Geometry check sheet. Reference: the model listing, model coordinates, mm. Face numbers are marked on the shaded views. A direction names the side the tool comes from. Give positions to 0.01 mm unless a question says otherwise; leave off trailing zeros. Loops run counter-clockwise (first coordinate to the right, second up) from the corner with the lowest first, then second, coordinate; pieces in that order, holes last. Notation, with made-up numbers: (36, -38.75) -> (75, -38.75) arc R24 cw to (75, -1.75) -> close; hole circle Ø3 at (-8, 68.5). An arc over 180 degrees is marked (long way). One line per question, with ' | ' between items.
from build123d import *

# Parameters (mm, degrees)
SKETCH_1_W           = 50
SKETCH_1_H           = 40
EXTRUDE_1_DEPTH      = 4
SKETCH_2_R           = 2
CUT_EXTRUDE_1_DEPTH  = 4
EXTRUDE_2_DEPTH      = 180
CUT_EXTRUDE_START    = -60
CUT_EXTRUDE_2_DEPTH  = 60
CUT_EXTRUDE_3_DEPTH  = 60
EXTRUDE_3_REACH      = 191.95
EXTRUDE_3_END_RADIUS = 230
EXTRUDE_START        = 38
EXTRUDE_4_DEPTH      = 38
CUT_EXTRUDE_4_DEPTH  = 211.154705038
SKETCH_9_R           = 3.5
EXTRUDE_5_DEPTH      = 40
SKETCH_10_R          = 1.5
CUT_EXTRUDE_5_DEPTH  = 30
CHAMFER_1_SIZE       = 0.5
EXTRUDE_6_REACH      = 171.111
EXTRUDE_6_END_RADIUS = 235
EXTRUDE_7_REACH      = 171.111


with BuildPart() as part:
    # 草图1 → 凸台-拉伸1 (new body)
    with BuildSketch(Plane(origin=(0, 0, 0), x_dir=(0, 0, -1), z_dir=(1, 0, 0))):
        with Locations((0, -20)):
            Rectangle(SKETCH_1_W, SKETCH_1_H)
    extrude(amount=EXTRUDE_1_DEPTH)

    # 草图2 → 切除-拉伸1 (cut)
    with BuildSketch(Plane(origin=(4, 0, 0), x_dir=(0, 0, -1), z_dir=(1, 0, 0))):
        with Locations((-15, -10)):
            Circle(SKETCH_2_R)
        with Locations((15, -10)):
            Circle(SKETCH_2_R)
    extrude(amount=-CUT_EXTRUDE_1_DEPTH, mode=Mode.SUBTRACT)

    # 草图3 → 凸台-拉伸2 (add)
    with BuildSketch(Plane(origin=(4, 0, 0), x_dir=(0, 0, -1), z_dir=(1, 0, 0))):
        with BuildLine():
            Line((-25, -33.637267303), (-25, -38.666428911))
            ThreePointArc((-25, -38.666428911), (0, -40), (25, -38.666428911))
            Line((25, -38.666428911), (25, -33.637267303))
            ThreePointArc((25, -33.637267303), (0, -35), (-25, -33.637267303))
        make_face()
    extrude(amount=EXTRUDE_2_DEPTH)

    # 草图4 → 切除-拉伸2 (cut)
    with BuildSketch(Plane(origin=(4, 0, 0), x_dir=(0, 0, -1), z_dir=(1, 0, 0)).offset(CUT_EXTRUDE_START)):
        with BuildLine():
            Line((25, -40), (25, -38.666428911))
            ThreePointArc((25, -38.666428911), (12.517771485, -39.666370401), (0, -40))
            Line((0, -40), (25, -40))
        make_face()
    extrude(amount=CUT_EXTRUDE_2_DEPTH, mode=Mode.SUBTRACT)

    # 草图5 → 切除-拉伸3 (cut)
    with BuildSketch(Plane(origin=(4, 0, 0), x_dir=(0, 0, -1), z_dir=(1, 0, 0)).offset(CUT_EXTRUDE_START)):
        with BuildLine():
            Line((-25, -38.666428911), (-25, -40))
            Line((-25, -40), (0, -40))
            ThreePointArc((0, -40), (-12.517771485, -39.666370401), (-25, -38.666428911))
        make_face()
    extrude(amount=CUT_EXTRUDE_3_DEPTH, mode=Mode.SUBTRACT)

    # 凸台-拉伸3: up to this cylinder (the profile starts outside it)
    extrude_3_end = Plane(origin=(65.000728, 195, 0), z_dir=(-1, 0, 0)) * Cylinder(EXTRUDE_3_END_RADIUS, 844.9, mode=Mode.PRIVATE)
    # 草图6 → 凸台-拉伸3 (add, up to the surface)
    with BuildSketch(Plane(origin=(0, -40, 0), x_dir=(-1, 0, 0), z_dir=(0, -1, 0)), mode=Mode.PRIVATE) as extrude_3_sk1:
        with BuildLine():
            Line((-85.002334196, 61.845829501), (-85.002334196, 25))
            Line((-85.002334196, 25), (-125, 25))
            ThreePointArc((-125, 25), (-130, 0), (-125, -25))
            Line((-125, -25), (-85.002334196, -25))
            Line((-85.002334196, -25), (-85.002334196, -61.845829501))
            ThreePointArc((-85.002334196, -61.845829501), (-65.002453212, -64.999999954), (-45.002334196, -61.84733917))
            Line((-45.002334196, -61.84733917), (-45.002334196, -25))
            Line((-45.002334196, -25), (-5, -25))
            ThreePointArc((-5, -25), (0, 0), (-5, 25))
            Line((-5, 25), (-45.002334196, 25))
            Line((-45.002334196, 25), (-45.002334196, 61.84733917))
            ThreePointArc((-45.002334196, 61.84733917), (-65.002453212, 64.999999954), (-85.002334196, 61.845829501))
        make_face()
    extrude_3_tool1 = extrude(extrude_3_sk1.sketch, amount=-EXTRUDE_3_REACH, mode=Mode.PRIVATE) - extrude_3_end
    extrude_3 = extrude_3_tool1.solids().sort_by_distance((65.000728, -40, 0))[0]
    add(extrude_3)

    # 镜向1: 凸台-拉伸3 across plane
    add(extrude_3.mirror(Plane.XY))

    # 草图7 → 凸台-拉伸4 (add)
    with BuildSketch(Plane.XZ.offset(40).offset(EXTRUDE_START)):
        with BuildLine():
            Line((5, -25), (8.810588186, -25))
            ThreePointArc((8.810588186, -25), (3.5, 0), (8.810588186, 25))
            Line((8.810588186, 25), (5, 25))
            ThreePointArc((5, 25), (1.26225608, 12.747548784), (0, 0))
            ThreePointArc((0, 0), (1.26225608, -12.747548784), (5, -25))
        make_face()
        with BuildLine():
            Line((45.002334196, -58.157917452), (45.002334196, -61.84733917))
            ThreePointArc((45.002334196, -61.84733917), (65.002453212, -64.999999954), (85.002334196, -61.845829501))
            Line((85.002334196, -61.845829501), (85.002334196, -58.156312011))
            ThreePointArc((85.002334196, -58.156312011), (65.002468367, -61.49999995), (45.002334196, -58.157917452))
        make_face()
        with BuildLine():
            Line((121.189411814, -25), (125, -25))
            ThreePointArc((125, -25), (128.73774392, -12.747548784), (130, 0))
            ThreePointArc((130, 0), (128.73774392, 12.747548784), (125, 25))
            Line((125, 25), (121.189411814, 25))
            ThreePointArc((121.189411814, 25), (126.5, 0), (121.189411814, -25))
        make_face()
        with BuildLine():
            Line((85.002334196, 58.156312011), (85.002334196, 61.845829501))
            ThreePointArc((85.002334196, 61.845829501), (65.002453212, 64.999999954), (45.002334196, 61.84733917))
            Line((45.002334196, 61.84733917), (45.002334196, 58.157917452))
            ThreePointArc((45.002334196, 58.157917452), (65.002468367, 61.49999995), (85.002334196, 58.156312011))
        make_face()
    extrude(amount=-EXTRUDE_4_DEPTH)

    # 草图8 → 切除-拉伸4 (cut, through all)
    with BuildSketch(Plane.XZ.offset(78)):
        with BuildLine():
            Line((184, 25), (125, 25))
            ThreePointArc((125, 25), (130, 0), (125, -25))
            Line((125, -25), (184, -25))
            Line((184, -25), (184, 25))
        make_face()
    extrude(amount=-CUT_EXTRUDE_4_DEPTH, mode=Mode.SUBTRACT)

    # 草图9 → 凸台-拉伸5 (add)
    with BuildSketch(Plane.XZ.offset(78)):
        with Locations((130, 0)):
            Circle(SKETCH_9_R)
        with Locations((65.002453212, -64.999999954)):
            Circle(SKETCH_9_R)
        with Locations((65.002453212, 64.999999954)):
            Circle(SKETCH_9_R)
    extrude(amount=-EXTRUDE_5_DEPTH)

    # 草图10 → 切除-拉伸5 (cut)
    with BuildSketch(Plane.XZ.offset(78)):
        with Locations(Location((65.002453212, 64.999999954, 0), (0, 0, 270))):
            Circle(SKETCH_10_R)
        with Locations(Location((130, 0, 0), (0, 0, 270))):
            Circle(SKETCH_10_R)
        with Locations(Location((65.002453212, -64.999999954, 0), (0, 0, 270))):
            Circle(SKETCH_10_R)
    extrude(amount=-CUT_EXTRUDE_5_DEPTH, mode=Mode.SUBTRACT)

    # 倒角1
    chamfer_1_edges = [part.edges().sort_by_distance(p)[0] for p in [
        (65.002453212, -78, 66.499999954),
        (130, -78, 1.5),
        (65.002453212, -78, -63.499999954),
    ]]
    chamfer(chamfer_1_edges, length=CHAMFER_1_SIZE)

    # 凸台-拉伸6: up to this cylinder (the profile starts outside it)
    extrude_6_end = Plane(origin=(1.489564, 195, 0), z_dir=(-1, 0, 0)) * Cylinder(EXTRUDE_6_END_RADIUS, 813.222, mode=Mode.PRIVATE)
    # 草图11 → 凸台-拉伸6 (add, up to the surface)
    with BuildSketch(Plane.XZ.offset(78), mode=Mode.PRIVATE) as extrude_6_sk1:
        with BuildLine():
            Line((0, 25), (0, 0))
            ThreePointArc((0, 0), (1.26225608, 12.747548784), (5, 25))
            Line((5, 25), (0, 25))
        make_face()
    extrude_6_tool1 = extrude(extrude_6_sk1.sketch, amount=-EXTRUDE_6_REACH, mode=Mode.PRIVATE) - extrude_6_end
    add(extrude_6_tool1.solids().sort_by_distance((1.489564, -78, 18.799089))[0])

    # 草图12 → 凸台-拉伸7 (add, up to next)
    with BuildSketch(Plane.XZ.offset(78), mode=Mode.PRIVATE) as extrude_7_sk1:
        with BuildLine():
            Line((0, -25), (5, -25))
            ThreePointArc((5, -25), (1.26225608, -12.747548784), (0, 0))
            Line((0, 0), (0, -25))
        make_face()
    extrude_7_tool1 = extrude(extrude_7_sk1.sketch, amount=-EXTRUDE_7_REACH, mode=Mode.PRIVATE) - part.part
    add(extrude_7_tool1.solids().sort_by_distance((1.489564, -78, -18.799089))[0])


solid = part.part
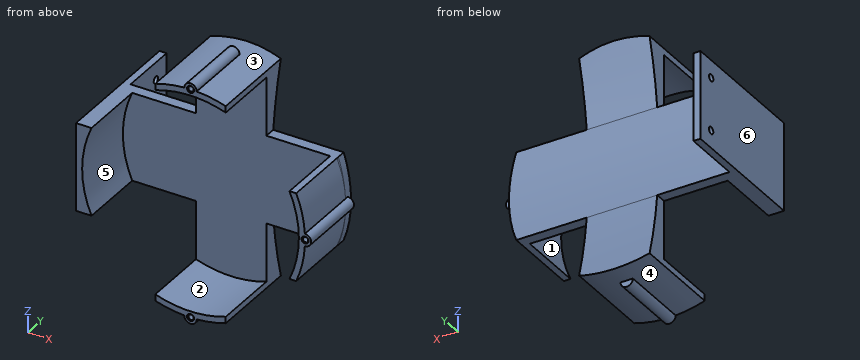
Item 1: Depth check by flat-ended pin: pin 1 Ø5 at (x, z) = (55.5, -40.5) entering from +Y; pin 2 Ø1.5 at (y, z) = (-21.5, -5) entering from +X; pin 3 Ø13.5 at (x, y) = (26, -26.5) entering from -Z; pin 4 Ø5 at (y, z) = (-35.5, 53) entering from -X. Enter the tip coordinate at first touch or a pass-through.
Result:
pin 1: y = -30.94 | pin 2: x = 4 | pin 3: through | pin 4: x = 45
Item 2: Scan lines: probe 1 along Y at (x, z) = (2.6, -15); probe 2 along Z at (x, y) = (130, -71.5); probe 3 along X at (y, z) = (-64, 0). Record each from-to range of solid material in increasing order.
Result:
probe 1: -78 to -12, -8 to 0 | probe 2: -3.5 to -1.5, 1.5 to 3.5 | probe 3: 0 to 3.5, 126.5 to 128.5, 131.5 to 133.5
Item 3: Sectioned sample at C-C (x = 47). Record the cut outline in (y, z).
Result:
outline: (-78, -62.46) -> (-26.36, -62.46) arc R230 cw to (-26.36, 62.46) -> (-78, 62.46) -> (-78, 58.81) -> (-40, 58.81) -> (-40, -58.81) -> (-78, -58.81) -> close
Item 4: Sectioned sample at D-D (z = 20). Record the cut outline in (x, y).
Result:
outline: (0, -78) -> (6.84, -78) -> (6.84, -40) -> (123.16, -40) -> (123.16, -78) -> (126.85, -78) -> (126.85, -34.13) -> (4, -34.13) -> (4, 0) -> (0, 0) -> close
Item 5: Sectioned sample at B-B (z = -15). Record the cut outline in (x, y), plus the area to 3 significant figures.
Result:
outline: (0, -78) -> (5.36, -78) -> (5.36, -40) -> (124.64, -40) -> (124.64, -78) -> (128.25, -78) -> (128.25, -34.51) -> (4, -34.51) -> (4, -12) -> (0, -12) -> close; (0, -8) -> (4, -8) -> (4, 0) -> (0, 0) -> close | area: 1,170 mm2
Item 6: Sectioned sample at A-A (y = -10). Record the cut outline in (x, z).
Result:
outline: (0, -25) -> (4, -25) -> (4, -17) -> (0, -17) -> close; (0, -13) -> (4, -13) -> (4, 13) -> (0, 13) -> close; (0, 17) -> (4, 17) -> (4, 25) -> (0, 25) -> close
Item 7: Release check for a two-part mould opening along Z. For the marked faces 1, 2, 3 and 4 record: pulls with the +Z half, pulls with the -Z half, needs draft (parallel to the pull), parting line crosses it, or undercut.
Result:
face 1: undercut | face 2: undercut | face 3: pulls with the +Z half | face 4: pulls with the -Z half
Item 8: Set-up check for the marked faces 5 and 6: record each of +Z, -Z, +X, -X, +Y, -Y from which the full face is reachable in a straight line by a thin tool's end or side.
Result:
face 5: -Y | face 6: +Z, -Z, -X, +Y, -Y
